Check sheet for the modelled part. Datum: model origin and axes. Units: mm. A direction names the side the tool comes from. Coordinates: 2 decimals unless noted, no trailing zeros. Order: outer loops, then holes, each group sorted by start corner. A loop starts at its lowest first (then second) coordinate and runs counter-clockwise, first axis right, second up.
1. Cross-section at B-B (y = 0). Enter the section's corners in (x, z), then the cut area to 3 significant figures.
2. Cross-section at D-D (z = 2.25). Enter the section's corners in (x, y).
3. Gauge pin test, flat ends, axial feed: pin 1 Ø6.5 at (x, z) = (16.06, 3.5) entering from +Y; pin 2 Ø6 at (y, z) = (-4, 8) entering from -X; pin 3 Ø5 at (y, z) = (-9, -2) entering from +X; pin 4 Ø1.5 at (x, y) = (12, -5.5) entering from -Z. Record the tip position at first contact, or that the pin passes through.
4. Draft check along Z on faces 1 (the flat face through (4, -4, 0)), 2 (the cylindrical face through (-10, 0, 5)), 3 (the cylindrical face through (20.06, -2.18, 3.67)). Enter one of: released by +Z, released by -Z, zero draft, split by the parting line, or undercut.
5. Set-up check for faces 4 (the flat face through (13, -25, 7)), 5 (the flat face through (6, -2, 4)), 6 (the flat face through (4, -4, 7)): record each of +Z, -Z, +X, -X, +Y, -Y from which the full face is reachable in a straight line by a thin tool's end or side.
6. Cross-section at C-C (x = 3). Enter the section's corners in (y, z).
7. Cross-section at A-A (z = 5.75). Enter the section's corners in (x, y), then the cut area to 3 significant figures.
8. Thickness scan on line 1 (X direction, y = -2.5, z = 1.25); line 2 (Z direction, x = 9.5, y = -4); line 3 (X direction, y = 2, z = 1.75). Record the ranges inside material, lowest first.
```python
from build123d import *

# Parameters (mm, degrees)
SKETCH_1_R           = 10
EXTRUDE_1_DEPTH      = 7
EXTRUDE_2_DEPTH      = 20
EXTRUDE_2_DEPTH_BACK = 25
SKETCH_2_R           = 7
SKETCH_3_R           = 4
SKETCH_3_W           = 26.062177826
SKETCH_3_H           = 1
CUT_EXTRUDE_1_DEPTH  = 55
SKETCH_4_R           = 5
CUT_EXTRUDE_2_DEPTH  = 55


with BuildPart() as part:
    # Эскиз1 → Бобышка-Вытянуть1 (new body)
    with BuildSketch(Plane.XY):
        Circle(SKETCH_1_R)
        with BuildLine():
            Line((10, -17.320508076), (10, 0))
            ThreePointArc((10, 0), (5, -8.660254038), (-5, -8.660254038))
            Line((-5, -8.660254038), (10, -17.320508076))
        make_face()
        with BuildLine():
            Line((10, 17.320508076), (-5, 8.660254038))
            ThreePointArc((-5, 8.660254038), (5, 8.660254038), (10, 0))
            Line((10, 0), (10, 17.320508076))
        make_face()
    extrude(amount=EXTRUDE_1_DEPTH)

    # Эскиз2 → Бобышка-Вытянуть2 (add, two sides: drawn at the far end of the back side and taken through both)
    with BuildSketch(Plane(origin=(0, 0, 0), x_dir=(1, 0, 0), z_dir=(0, 1, 0)).offset(-EXTRUDE_2_DEPTH_BACK)):
        with Locations(Location((16.062177826, -3.5, 0), (0, 0, 270))):
            Circle(SKETCH_2_R)
    extrude(amount=EXTRUDE_2_DEPTH + EXTRUDE_2_DEPTH_BACK)

    # Эскиз3 → Вырез-Вытянуть1 (cut)
    with BuildSketch(Plane(origin=(0, 20, 0), x_dir=(1, 0, 0), z_dir=(0, 1, 0))):
        with Locations((16.062177826, -3.5)):
            Circle(SKETCH_3_R)
        with Locations((3.031088913, -3.5)):
            Rectangle(SKETCH_3_W, SKETCH_3_H)
    extrude(amount=-CUT_EXTRUDE_1_DEPTH, mode=Mode.SUBTRACT)

    # Эскиз4 → Вырез-Вытянуть2 (cut)
    with BuildSketch(Plane.XY.offset(7)):
        Circle(SKETCH_4_R)
    extrude(amount=-CUT_EXTRUDE_2_DEPTH, mode=Mode.SUBTRACT)


solid = part.part
```
Data:
1. outline: (-10, 0) - (-5, 0) - (-5, 3) - (-10, 3) - close; (-10, 4) - (-5, 4) - (-5, 7) - (-10, 7) - close; (5, 0) - (10, 0) arc R7 ccw (long way) to (10, 7) - (5, 7) - (5, 4) - (12.09, 4) arc R4 cw (long way) to (12.09, 3) - (5, 3) - close
1. area: 157 mm2
2. outline: (-5, -8.66) - (9.17, -16.84) - (9.17, -25) - (12.26, -25) - (12.26, 20) - (9.17, 20) - (9.17, 16.84) - (-5, 8.66) arc R10 ccw to start; (19.86, -25) - (22.95, -25) - (22.95, 20) - (19.86, 20) - close; hole circle Ø10 at (0, 0)
3. pin 1: passes through
3. pin 2: stops at x = -9.93
3. pin 3: stops at x = 22.39
3. pin 4: stops at z = -2.67
4. face 1: released by -Z
4. face 2: zero draft
4. face 3: undercut
5. face 4: +Z, -Z, +X, -X, -Y
5. face 5: -X, +Y, -Y
5. face 6: +Z, -X, +Y, -Y
6. outline: (-13.28, 0) - (-4, 0) - (-4, 3) - (-13.28, 3) - close; (-13.28, 4) - (-4, 4) - (-4, 7) - (-13.28, 7) - close; (4, 0) - (13.28, 0) - (13.28, 3) - (4, 3) - close; (4, 4) - (13.28, 4) - (13.28, 7) - (4, 7) - close
7. outline: (-5, -8.66) - (9.43, -16.99) - (9.43, -25) - (12.75, -25) - (12.75, 20) - (9.43, 20) - (9.43, 16.99) - (-5, 8.66) arc R10 ccw to start; (19.37, -25) - (22.69, -25) - (22.69, 20) - (19.37, 20) - close; hole circle Ø10 at (0, 0)
7. area: 652 mm2
8. line 1: x = -9.68 to -4.33, 4.33 to 12.75, 19.37 to 22.69
8. line 2: z = 0 to 3, 4 to 7
8. line 3: x = -9.8 to -4.58, 4.58 to 12.47, 19.66 to 22.84
